Verification items for this drawing (mm, ordinates from the low corner). A direction names the side the tool comes from. Give positions to 0.01 mm unless a question says otherwise; leave off trailing zeros. Write each loop counter-clockwise with the first axis right and the second up, starting at its lowest first coordinate (ties: lowest second). Pieces come first, ordered by that corner, then holes. Notation, with made-up numbers: (11, 11) -> (48, 11) arc R6 cw to (48, 21) -> close; hole circle Ø2 at (-15, 50.5). An arc over 180 degrees is marked (long way). Write item = value, one per line.
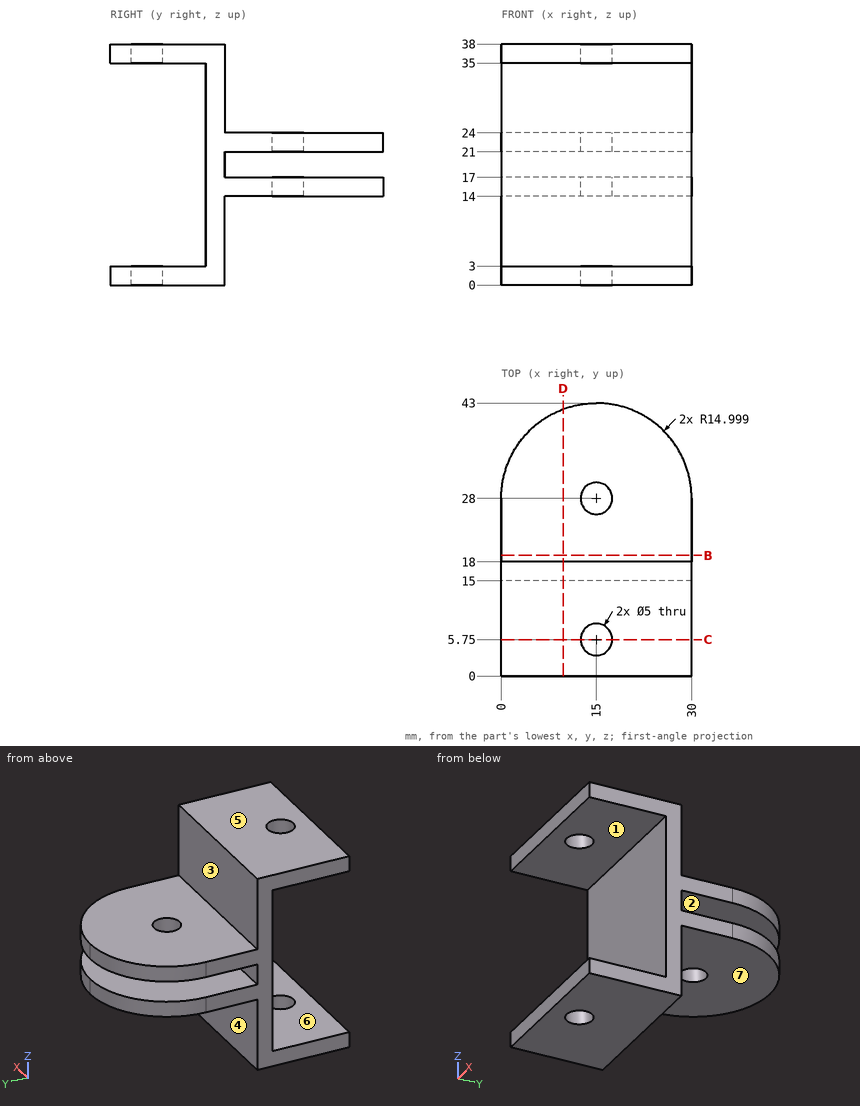
Item 1: Go/stop test with flat-tipped pins: P1, Ø10, axis at x = 4.5, y = 35, coming from the +Z side; P2, Ø15, axis at x = 8.5, z = 13.5, coming from the -Y side; P3, Ø10, axis at y = 35.5, z = 22.5, coming from the +X side; P4, Ø4.5, axis at x = 15, y = 28, coming from the -Z side. Record where each tip stops, or that it passes through.
Response values:
P1 = 24
P2 = 15
P3 = 29.79
P4 = through
Item 2: Sectioned sample at B-B on y = 19. Record the cut outline in (x, z).
Response values:
outline = (0, 14) -> (30, 14) -> (30, 17) -> (0, 17) -> close; (0, 21) -> (30, 21) -> (30, 24) -> (0, 24) -> close
Item 3: Mould release check, pull along Z, two halves, no side actions. Record for the marked faces 5, 6 and 7: +Z half, -Z half, draft (parallel to the pull), parting line (faces both ways), or undercut.
Response values:
face_5 = +Z half
face_6 = undercut
face_7 = -Z half
Item 4: Set-up check for the marked faces 1, 2, 3 and 4: record each of +Z, -Z, +X, -X, +Y, -Y from which the full face is reachable in a straight line by a thin tool's end or side.
Response values:
face_1 = +X, -X, -Y
face_2 = +X, -X, +Y
face_3 = +Z, +X, -X, +Y
face_4 = -Z, +X, -X, +Y
Item 5: Sectioned sample at C-C on y = 5.75. Record the cut outline in (x, z), then the cut area to 3 significant figures.
Response values:
outline = (0, 0) -> (12.5, 0) -> (12.5, 3) -> (0, 3) -> close; (0, 35) -> (12.5, 35) -> (12.5, 38) -> (0, 38) -> close; (17.5, 0) -> (30, 0) -> (30, 3) -> (17.5, 3) -> close; (17.5, 35) -> (30, 35) -> (30, 38) -> (17.5, 38) -> close
area = 150 mm^2
Item 6: Sectioned sample at D-D on x = 9.75. Record the cut outline in (y, z).
Response values:
outline = (0, 0) -> (18, 0) -> (18, 14) -> (42.05, 14) -> (42.05, 17) -> (18, 17) -> (18, 21) -> (42.05, 21) -> (42.05, 24) -> (18, 24) -> (18, 38) -> (0, 38) -> (0, 35) -> (15, 35) -> (15, 3) -> (0, 3) -> close
Item 7: Material ranges on line 1 (Y direction, x = 15, z = 23.3); line 2 (X direction, y = 28, z = 23); line 3 (Z direction, x = 14.5, y = 33), recorded low to high.
Response values:
line_1 = 15 to 25.5, 30.5 to 43
line_2 = 0 to 12.5, 17.5 to 30
line_3 = 14 to 17, 21 to 24
